Check sheet for the modelled part. Datum: model origin and axes. Units: mm. A direction names the side the tool comes from. Coordinates: 2 decimals unless noted, no trailing zeros. Order: outer loops, then holes, each group sorted by start corner. A loop starts at its lowest first (then second) coordinate and runs counter-clockwise, first axis right, second up.
from build123d import *

# Parameters (mm, degrees)
F0_W      = 53.264
F0_H      = 92
F1_DEPTH  = 12.7
F2_W      = 53.264
F2_H      = 19.05
F3_DEPTH  = 6.35
F4_W      = 53.264
F4_H      = 19.05
F5_DEPTH  = 6.35
F6_DEPTH  = 1.15
F7_D      = 6.528
F8_W      = 39.264
F8_H      = 13
F9_DEPTH  = 13.851
F10_W     = 32
F10_H     = 7.5
F11_DEPTH = 3


with BuildPart() as f1:
    # F0 (on Top) → F1 (new body)
    with BuildSketch(Plane.XY):
        with Locations((3.9193365263, 5.0369417648)):
            Rectangle(F0_W, F0_H)
    extrude(amount=F1_DEPTH)

    # F2 (on face) → F3 (cut)
    with BuildSketch(Plane(origin=(0, 0, 0), x_dir=(1, 0, 0), z_dir=(0, 0, -1))):
        with Locations((3.9193365263, -41.5119417648)):
            Rectangle(F2_W, F2_H)
    extrude(amount=-F3_DEPTH, mode=Mode.SUBTRACT)

    # F4 (on face) → F5 (cut)
    with BuildSketch(Plane.XY.offset(12.7)):
        with Locations((3.9193365263, -31.4380582352)):
            Rectangle(F4_W, F4_H)
    extrude(amount=-F5_DEPTH, mode=Mode.SUBTRACT)

    # F6 (add): a face of the model
    f6_faces = [f1.faces().sort_by_distance(p)[0] for p in [
        (3.9193365263, 14.5619417648, 12.7),
    ]]
    extrude(f6_faces, amount=F6_DEPTH)

    # F7 (through all)
    with Locations(Plane(origin=(0, 0, 0), x_dir=(1, 0, 0), z_dir=(0, 0, -1))):
        with Locations((-14.8366634737, 31.4380582352), (22.6753365263, 31.4380582352), (-14.8366634737, -41.6389417648), (22.6753365263, -41.6389417648)):
            Hole(F7_D / 2)

    # F8 (on face) → F9 (cut, through all)
    with BuildSketch(Plane(origin=(0, 0, 0), x_dir=(1, 0, 0), z_dir=(0, 0, -1))):
        with Locations((3.9193365263, 4.4630582352)):
            Rectangle(F8_W, F8_H)
        with Locations((3.9193365263, -18.4869417648)):
            Rectangle(F8_W, F8_H)
    extrude(amount=-F9_DEPTH, mode=Mode.SUBTRACT)

    # F10 (on face) → F11 (cut)
    with BuildSketch(Plane.XZ.offset(21.9130582352)):
        with Locations((3.9193365263, 10.1)):
            Rectangle(F10_W, F10_H)
    extrude(amount=-F11_DEPTH, mode=Mode.SUBTRACT)


solid = f1.part
(1) Go/stop test with flat-tipped pins: P1, Ø8, axis at x = 23.5, z = 11, coming from the -Y side; P2, Ø1.9, axis at x = 12.5, z = 2.5, coming from the +Y side; P3, Ø11, axis at x = -1.5, y = -34, coming from the +Z side. Record where each tip stops, or that it passes through.
Filled in:
P1: stops at y = -21.91
P2: stops at y = 31.99
P3: stops at z = 6.35
(2) Release check for a two-part mould opening along X. For faces 1 (the flat face through (4, 7, 13.85)), 2 (the flat face through (23.551, -4, 7)), 3 (the flat face through (30.551, 4, 7)) record: +X half, -X half, draft (parallel to the pull), parting line (faces both ways), or undercut.
Filled in:
face 1: draft
face 2: undercut
face 3: +X half
(3) Tool access check on faces 4 (the flat face through (19.919, -20, 10)), 5 (the flat face through (4, -12, 0)), 6 (the flat face through (4, 31.987, 3)), 7 (the flat face through (-17, -21.913, 10)), 8 (the flat face through (23.551, 19, 7)). Record the directions out of +Z, -Z, +X, -X, +Y, -Y that give a thin tool (end or side, any length) a straight path to the whole face; none if there is none.
Filled in:
face 4: +Z, -Y
face 5: -Z, +X, -X, +Y, -Y
face 6: -Z, +X, -X, +Y
face 7: +Z, +X, -X, -Y
face 8: +Z, -Z
(4) Cross-section at B-B (y = 0). Enter the section's corners in (x, z).
Filled in:
outline: (-22.71, 0) - (-15.71, 0) - (-15.71, 13.85) - (-22.71, 13.85) - close; (23.55, 0) - (30.55, 0) - (30.55, 13.85) - (23.55, 13.85) - close
(5) Cross-section at C-C (y = -33.5). Enter the section's corners in (x, z).
Filled in:
outline: (-22.71, 0) - (-17.37, 0) - (-17.37, 6.35) - (-22.71, 6.35) - close; (-12.31, 0) - (20.15, 0) - (20.15, 6.35) - (-12.31, 6.35) - close; (25.21, 0) - (30.55, 0) - (30.55, 6.35) - (25.21, 6.35) - close
(6) Cross-section at A-A (x = 18.5). Enter the section's corners in (y, z).
Filled in:
outline: (-40.96, 0) - (-10.96, 0) - (-10.96, 13.85) - (-18.91, 13.85) - (-18.91, 6.35) - (-40.96, 6.35) - close; (2.04, 0) - (11.99, 0) - (11.99, 13.85) - (2.04, 13.85) - close; (24.99, 0) - (31.99, 0) - (31.99, 6.35) - (51.04, 6.35) - (51.04, 13.85) - (24.99, 13.85) - close
(7) Cross-section at D-D (z = 4). Enter the section's corners in (x, y), and give its area (3 significant figures).
Filled in:
outline: (-22.71, -40.96) - (30.55, -40.96) - (30.55, 31.99) - (-22.71, 31.99) - close; hole circle Ø6.53 at (-14.84, -31.44); hole (-15.71, -10.96) - (23.55, -10.96) - (23.55, 2.04) - (-15.71, 2.04) - close; hole (-15.71, 11.99) - (23.55, 11.99) - (23.55, 24.99) - (-15.71, 24.99) - close; hole circle Ø6.53 at (22.68, -31.44)
area: 2,800 mm2
(8) Thickness scan on probe 1 along Y at (x, z) = (17, 7.75); probe 2 along Y at (x, z) = (-11, 5.25); probe 3 along Y at (x, z) = (23, 3.75). Record the ranges inside material, lowest first.
Filled in:
probe 1: y = -18.91 to -10.96, 2.04 to 11.99, 24.99 to 51.04
probe 2: y = -40.96 to -10.96, 2.04 to 11.99, 24.99 to 31.99
probe 3: y = -40.96 to -34.69, -28.19 to -10.96, 2.04 to 11.99, 24.99 to 31.99
